The model under review builds one solid part; all positions refer to its coordinate system, in mm. Face numbers are marked on the shaded views. A direction names the side the tool comes from. Round coordinates to 2 decimals unless told otherwise and drop trailing zeros. Order: outer loops, then holes, each group sorted by start corner. A loop starts at its lowest first (then second) coordinate and runs counter-clockwise, first axis right, second up.
```python
from build123d import *

# Parameters (mm, degrees)
BASE_EXTRUDE_THIN_DEPTH = 19.05
CUT_EXTRUDE1_REACH      = 97.25
SKETCH2_R               = 6.35


with BuildPart() as part:
    # Sketch1 → Base-Extrude-Thin (new body, symmetric)
    with BuildSketch(Plane(origin=(0, 0, 0), x_dir=(0, 0, -1), z_dir=(1, 0, 0))):
        with BuildLine():
            Line((-62.443024211, 21.3868), (-26.136761314, 0.425369343))
            ThreePointArc((-26.136761314, 0.425369343), (-25.371011782, 0.108185502), (-24.549261314, 0))
            Line((-24.549261314, 0), (-3.175, 0))
            ThreePointArc((-3.175, 0), (-0.92993597, 0.92993597), (0, 3.175))
            Line((0, 3.175), (0, 79.375))
            ThreePointArc((0, 79.375), (-0.92993597, 81.62006403), (-3.175, 82.55))
            Line((-3.175, 82.55), (-44.45, 82.55))
            Line((-44.45, 82.55), (-44.45, 88.9))
            Line((-44.45, 88.9), (-3.175, 88.9))
            ThreePointArc((-3.175, 88.9), (3.560192091, 86.110192091), (6.35, 79.375))
            Line((6.35, 79.375), (6.35, 3.175))
            ThreePointArc((6.35, 3.175), (3.560192091, -3.560192091), (-3.175, -6.35))
            Line((-3.175, -6.35), (-24.549261314, -6.35))
            ThreePointArc((-24.549261314, -6.35), (-27.014512719, -6.025443495), (-29.311761314, -5.073891971))
            Line((-29.311761314, -5.073891971), (-65.618024211, 15.887538686))
            Line((-65.618024211, 15.887538686), (-62.443024211, 21.3868))
        make_face()
    extrude(amount=BASE_EXTRUDE_THIN_DEPTH, both=True)

    # Sketch2 → Cut-Extrude1 (cut, up to next)
    with BuildSketch(Plane(origin=(0, 88.9, 0), x_dir=(-1, 0, 0), z_dir=(0, 1, 0)), mode=Mode.PRIVATE) as cut_extrude1_sk1:
        with Locations((0, 25.4)):
            Circle(SKETCH2_R)
    cut_extrude1_tool1 = extrude(cut_extrude1_sk1.sketch, amount=-CUT_EXTRUDE1_REACH, mode=Mode.PRIVATE) & part.part
    add(cut_extrude1_tool1.solids().sort_by_distance((0, 88.9, 25.4))[0], mode=Mode.SUBTRACT)


solid = part.part
```
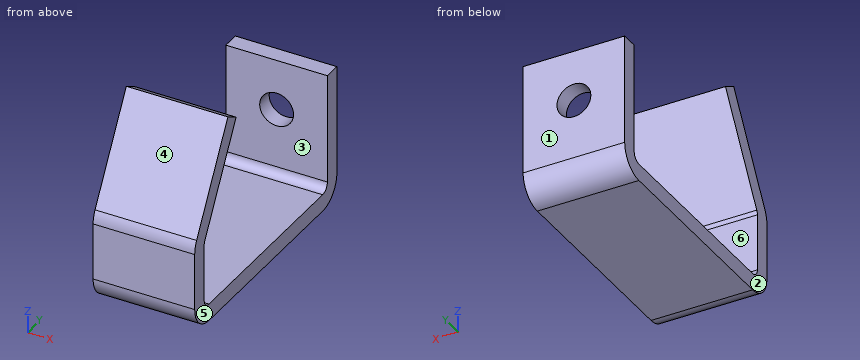
(1) To check wall thickness, follow probe 1 along X at (y, z) = (87, 25); probe 2 along Y at (x, z) = (17.5, 20.5); probe 3 along Z at (x, y) = (0, 84.5). State the ranges of each line that lie inside material, in increasing order.
Data:
probe 1: x = -19.05 to -6.34, 6.34 to 19.05
probe 2: y = -6.35 to 0, 82.55 to 88.9
probe 3: z = -4.85 to 19.05, 31.75 to 44.45
(2) Consider section D-D (y = 31). Write out the cut boundary in (x, z).
Data:
outline: (-19.05, -6.35) - (19.05, -6.35) - (19.05, 0) - (-19.05, 0) - close
(3) Insertion check: pin 1 (5 mm diameter, centred on x = -2, y = 85.5, fed in from +Z); pin 2 (8 mm diameter, centred on x = -13, y = 60, fed in from +Z). Each pin has a flat end and moves straight along its axis. Give the tip position at first contact, or say it passes through.
Data:
pin 1: stops at z = 44.45
pin 2: stops at z = 0
(4) Consider section B-B (x = 10). Write out the cut boundary in (y, z) (3 decimals), and give its area (3 significant figures).
Data:
outline: (-6.35, 3.175) arc R9.525 ccw to (3.175, -6.35) - (79.375, -6.35) arc R9.525 ccw to (88.9, 3.175) - (88.9, 44.45) - (82.55, 44.45) - (82.55, 3.175) arc R3.175 cw to (79.375, 0) - (3.175, 0) arc R3.175 cw to (0, 3.175) - (0, 24.549) arc R3.175 cw to (0.425, 26.137) - (21.387, 62.443) - (15.888, 65.618) - (-5.074, 29.312) arc R9.525 ccw to (-6.35, 24.549) - close
area: 1,300 mm2
(5) Consider section A-A (x = 0). Write out the cut boundary in (y, z) (3 decimals).
Data:
outline: (-6.35, 3.175) arc R9.525 ccw to (3.175, -6.35) - (79.375, -6.35) arc R9.525 ccw to (88.9, 3.175) - (88.9, 19.05) - (82.55, 19.05) - (82.55, 3.175) arc R3.175 cw to (79.375, 0) - (3.175, 0) arc R3.175 cw to (0, 3.175) - (0, 24.549) arc R3.175 cw to (0.425, 26.137) - (21.387, 62.443) - (15.888, 65.618) - (-5.074, 29.312) arc R9.525 ccw to (-6.35, 24.549) - close; (82.55, 31.75) - (88.9, 31.75) - (88.9, 44.45) - (82.55, 44.45) - close
(6) Draft analysis for pull direction Y (two halves, no side actions). For the marked faces 1, 2, 3 and 4, state which applies: pulls with the +Y half, pulls with the -Y half, needs draft (parallel to the pull), parting line crosses it, or undercut.
Data:
face 1: pulls with the +Y half
face 2: needs draft
face 3: undercut
face 4: pulls with the -Y half
(7) For the marked faces 5 and 6, list the 3-axis set-ups (+Z, -Z, +X, -X, +Y, -Y) from which the entire face can be reached by the end or side of a thin tool; tool diameter is ignored.
Data:
face 5: +Z, -Z, +X, +Y, -Y
face 6: +X, -X
(8) Consider section C-C (z = 21). Write out the cut boundary in (x, y), and give its area (3 significant figures).
Data:
outline: (-19.05, -6.35) - (19.05, -6.35) - (19.05, 0) - (-19.05, 0) - close; (-19.05, 82.55) - (-4.58, 82.55) - (-4.58, 88.9) - (-19.05, 88.9) - close; (4.58, 82.55) - (19.05, 82.55) - (19.05, 88.9) - (4.58, 88.9) - close
area: 426 mm2
